Model file for the job. Use its own axes, mm. Coordinates: 2 decimals unless noted, no trailing zeros. Order: outer loops, then holes, each group sorted by start corner. A loop starts at its lowest first (then second) coordinate and runs counter-clockwise, first axis right, second up. Notation, with made-up numbers: (64, 59.5) -> (76, 59.5) arc R23 cw to (76, 97.5) -> close; hole circle Ø6 at (-4.5, -9). An arc over 180 degrees is marked (long way). Write item = value, one per line. Start each with the question number.
Q1. Cut at B-B, the plane x = 70. List the corners of the cut face in (y, z), plus the area to 3 significant figures.
Q2. Cut at C-C, the plane y = 37.5. List the corners of the cut face in (x, z), plus the area to 3 significant figures.
Q3. Flat gauge pins, fed straight in: pin 1 (1.8 mm diameter, centred on x = 10, y = 10, fed in from +Z); pin 2 (2 mm diameter, centred on x = 5, z = 1.5, fed in from -Y); pin 3 (2 mm diameter, centred on x = -9, z = 2, fed in from +Y); pin 4 (2 mm diameter, centred on x = 73.5, z = 3, fed in from +Y). Where does each tip first touch, or does it go through?
Q4. Cut at D-D, the plane z = 1.9. Give the number of separate pieces and of enclosed holes in the cut face, plus the area to 3 significant figures.
Q5. Cut at A-A, the plane y = 85. List the corners of the cut face in (x, z), plus the area to 3 significant figures.
Q6. Wall check: line 1 (Y direction, x = 104.5, z = 2.2); line 2 (Y direction, x = -2.5, z = 2.25); line 3 (X direction, y = -1, z = 2.7). Give the ranges that are in metal, low to high. Write a range as from..to.
from build123d import *

# Parameters (mm, degrees)
F0_R     = 1.65
F0_R_2   = 2.55
F0_R_3   = 1.525
F0_W     = 5
F0_H     = 10
F0_R_4   = 3.555
F1_DEPTH = 4


with BuildPart() as f1:
    # F0 (on Top) → F1 (new body)
    with BuildSketch(Plane.XY):
        with BuildLine():
            ThreePointArc((-56.363239, 23.1312), (-55.348378, 20.999418), (-54.999976, 18.664241))
            Line((-54.999976, 18.664241), (-54.999976, -18.664242))
            ThreePointArc((-54.999976, -18.664242), (-55.348378, -20.999419), (-56.363239, -23.1312))
            Line((-56.363239, -23.1312), (-109.062757, -101.428966))
            ThreePointArc((-109.062757, -101.428966), (-108.056825, -108.695115), (-100.723998, -108.498976))
            Line((-100.723998, -108.498976), (-30.492366, -42.183308))
            ThreePointArc((-30.492366, -42.183308), (-27.955204, -40.565838), (-25, -40))
            Line((-25, -40), (25, -40))
            ThreePointArc((25, -40), (27.955204, -40.565838), (30.492367, -42.183308))
            Line((30.492367, -42.183308), (100.723998, -108.498976))
            ThreePointArc((100.723998, -108.498976), (108.056825, -108.695115), (109.062757, -101.428966))
            Line((109.062757, -101.428966), (56.363239, -23.1312))
            ThreePointArc((56.363239, -23.1312), (55.348379, -20.999418), (54.999977, -18.664242))
            Line((54.999977, -18.664242), (54.999977, 18.664241))
            ThreePointArc((54.999977, 18.664241), (55.348379, 20.999418), (56.363239, 23.1312))
            Line((56.363239, 23.1312), (109.062757, 101.428966))
            ThreePointArc((109.062757, 101.428966), (108.056825, 108.695115), (100.723998, 108.498976))
            Line((100.723998, 108.498976), (30.492367, 42.183307))
            ThreePointArc((30.492367, 42.183307), (27.955204, 40.565837), (25, 40))
            Line((25, 40), (-25, 40))
            ThreePointArc((-25, 40), (-27.955204, 40.565837), (-30.492366, 42.183307))
            Line((-30.492366, 42.183307), (-100.723998, 108.498976))
            ThreePointArc((-100.723998, 108.498976), (-108.056825, 108.695115), (-109.062757, 101.428966))
            Line((-109.062757, 101.428966), (-56.363239, 23.1312))
        make_face()
        with Locations((-104.5, -104.5)):
            Circle(F0_R, mode=Mode.SUBTRACT)
        with Locations((-87.96694, -85)):
            Circle(F0_R_2, mode=Mode.SUBTRACT)
        with Locations((-44.444976, -20.807752)):
            Circle(F0_R_2, mode=Mode.SUBTRACT)
        with BuildLine():
            ThreePointArc((-34, 14.278979), (-32.187663, 17.033876), (-28.940362, 16.460239))
            Line((-28.940362, 16.460239), (-13.818204, 2.181259))
            ThreePointArc((-13.818204, 2.181259), (-12.877841, -1e-06), (-13.818204, -2.18126))
            Line((-13.818204, -2.18126), (-28.940362, -16.460239))
            ThreePointArc((-28.940362, -16.460239), (-32.187663, -17.033877), (-34, -14.27898))
            Line((-34, -14.27898), (-34, 14.278979))
        make_face(mode=Mode.SUBTRACT)
        with Locations((-10, -10)):
            Circle(F0_R_3, mode=Mode.SUBTRACT)
        with Locations((104.5, -104.5)):
            Circle(F0_R, mode=Mode.SUBTRACT)
        with Locations((87.966941, -85)):
            Circle(F0_R_2, mode=Mode.SUBTRACT)
        with BuildLine():
            ThreePointArc((-14.278979, -34), (-17.06679, -32.108202), (-16.338617, -28.818741))
            Line((-16.338617, -28.818741), (-2.059637, -15.335926))
            ThreePointArc((-2.059637, -15.335926), (0, -14.517186), (2.059638, -15.335926))
            Line((2.059638, -15.335926), (16.338617, -28.818741))
            ThreePointArc((16.338617, -28.818741), (17.06679, -32.108202), (14.27898, -34))
            Line((14.27898, -34), (-14.278979, -34))
        make_face(mode=Mode.SUBTRACT)
        with Locations((10, -10)):
            Circle(F0_R_3, mode=Mode.SUBTRACT)
        with Locations((44.444977, -20.807752)):
            Circle(F0_R_2, mode=Mode.SUBTRACT)
        with Locations((-49.499976, 0)):
            Rectangle(F0_W, F0_H, mode=Mode.SUBTRACT)
        with Locations((-44.444976, 20.810818)):
            Circle(F0_R_4, mode=Mode.SUBTRACT)
        with Locations((-10, 10)):
            Circle(F0_R_3, mode=Mode.SUBTRACT)
        with Locations((-87.96694, 85)):
            Circle(F0_R_4, mode=Mode.SUBTRACT)
        with Locations((-104.5, 104.5)):
            Circle(F0_R, mode=Mode.SUBTRACT)
        with Locations((10, 10)):
            Circle(F0_R_3, mode=Mode.SUBTRACT)
        with BuildLine():
            ThreePointArc((28.940363, 16.460239), (32.187664, 17.033876), (34, 14.278979))
            Line((34, 14.278979), (34, -14.27898))
            ThreePointArc((34, -14.27898), (32.187663, -17.033876), (28.940363, -16.460239))
            Line((28.940363, -16.460239), (13.818205, -2.18126))
            ThreePointArc((13.818205, -2.18126), (12.877842, 0), (13.818205, 2.181259))
            Line((13.818205, 2.181259), (28.940363, 16.460239))
        make_face(mode=Mode.SUBTRACT)
        with BuildLine():
            ThreePointArc((14.27898, 34), (17.066791, 32.108201), (16.338617, 28.81874))
            Line((16.338617, 28.81874), (2.059638, 15.335925))
            ThreePointArc((2.059638, 15.335925), (0, 14.517185), (-2.059637, 15.335925))
            Line((-2.059637, 15.335925), (-16.338617, 28.81874))
            ThreePointArc((-16.338617, 28.81874), (-17.06679, 32.108201), (-14.278979, 34))
            Line((-14.278979, 34), (14.27898, 34))
        make_face(mode=Mode.SUBTRACT)
        with Locations((49.499977, 0)):
            Rectangle(F0_W, F0_H, mode=Mode.SUBTRACT)
        with Locations((44.444977, 20.810818)):
            Circle(F0_R_4, mode=Mode.SUBTRACT)
        with Locations((87.966941, 85)):
            Circle(F0_R_4, mode=Mode.SUBTRACT)
        with Locations((104.5, 104.5)):
            Circle(F0_R, mode=Mode.SUBTRACT)
    extrude(amount=F1_DEPTH)


solid = f1.part
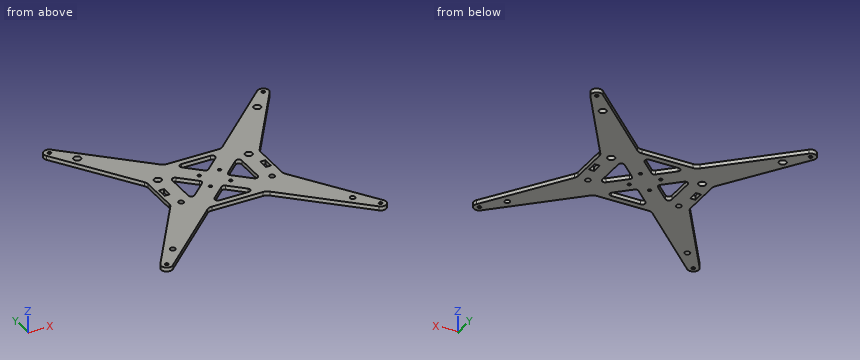
Here are the results:
q1.outline = (-79.49, 0) -> (-43.39, 0) -> (-43.39, 4) -> (-79.49, 4) -> close; (43.39, 0) -> (79.49, 0) -> (79.49, 4) -> (43.39, 4) -> close
q1.area = 289 mm²
q2.outline = (-66.03, 0) -> (66.03, 0) -> (66.03, 4) -> (-66.03, 4) -> close
q2.area = 528 mm²
q3.pin_1 = through
q3.pin_2 = -40
q3.pin_3 = 40
q3.pin_4 = 83.74
q4.separate_pieces = 1
q4.enclosed_holes = 22
q4.area = 14,300 mm²
q5.outline = (-98, 0) -> (-91.52, 0) -> (-91.52, 4) -> (-98, 4) -> close; (-84.41, 0) -> (-75.84, 0) -> (-75.84, 4) -> (-84.41, 4) -> close; (75.84, 0) -> (84.41, 0) -> (84.41, 4) -> (75.84, 4) -> close; (91.52, 0) -> (98, 0) -> (98, 4) -> (91.52, 4) -> close
q5.area = 120 mm²
q6.line_1 = -110..-106.15, -102.85..-94.65, 94.65..102.85, 106.15..110
q6.line_2 = -40..-34, -15.75..15.75, 34..40
q6.line_3 = -55..-52, -47..-34, -13.05..13.05, 34..47, 52..55
